CAD build for the part. Positions are in the model's coordinates, mm. Face numbers are marked on the shaded views. A direction names the side the tool comes from. Round coordinates to 2 decimals unless told otherwise and drop trailing zeros.
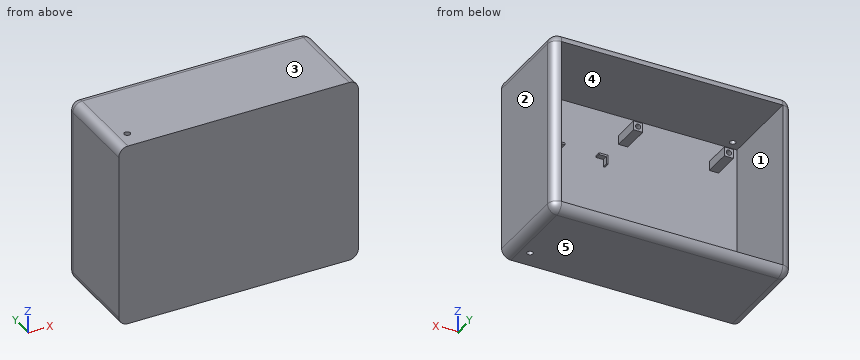
```python
from build123d import *

# Parameters (mm, degrees)
SKETCH1_W                                         = 130
SKETCH1_H                                         = 100
BOSS_EXTRUDE1_DEPTH                               = 51
SKETCH2_W                                         = 120
SKETCH2_H                                         = 90
CUT_EXTRUDE1_DEPTH                                = 46
FILLET2_R                                         = 5
FILLET4_R                                         = 5
SKETCH6_W                                         = 5
SKETCH6_H                                         = 5
BOSS_EXTRUDE2_DEPTH                               = 15
BOSS_EXTRUDE3_DEPTH                               = 3
F_4_CLEARANCE_HOLE2_D                             = 2.8448
F_4_CLEARANCE_HOLE2_DEPTH                         = 10
CSK_FOR_4_FLAT_HEAD_MACHINE_SCREW_100_D           = 3.2639
CSK_FOR_4_FLAT_HEAD_MACHINE_SCREW_100_DEPTH       = 10
CSK_FOR_4_FLAT_HEAD_MACHINE_SCREW_100_CSINK_D     = 5.715
CSK_FOR_4_FLAT_HEAD_MACHINE_SCREW_100_CSINK_ANGLE = 100
CSK_FOR_4_FLAT_HEAD_MACHINE_SCREW_100_TIP         = 0.980574487
CSK_FOR_4_FLAT_HEAD_MACHINE_SCREW_2_D             = 3.2639
CSK_FOR_4_FLAT_HEAD_MACHINE_SCREW_2_DEPTH         = 10
CSK_FOR_4_FLAT_HEAD_MACHINE_SCREW_2_CSINK_D       = 5.715
CSK_FOR_4_FLAT_HEAD_MACHINE_SCREW_2_CSINK_ANGLE   = 100
CSK_FOR_4_FLAT_HEAD_MACHINE_SCREW_2_TIP           = 0.980574487


# Some blends are built 0.0001 mm under size
with BuildPart() as part:
    # Sketch1 → Boss-Extrude1 (new body)
    with BuildSketch(Plane(origin=(0, 0, 0), x_dir=(1, 0, 0), z_dir=(0, 1, 0))):
        Rectangle(SKETCH1_W, SKETCH1_H)
    extrude(amount=BOSS_EXTRUDE1_DEPTH)

    # Sketch2 → Cut-Extrude1 (cut)
    with BuildSketch(Plane(origin=(0, 51, 0), x_dir=(1, 0, 0), z_dir=(0, 1, 0))):
        Rectangle(SKETCH2_W, SKETCH2_H)
    extrude(amount=-CUT_EXTRUDE1_DEPTH, mode=Mode.SUBTRACT)

    # Fillet2
    fillet2_edges = [part.edges().sort_by_distance(p)[0] for p in [
        (-65, 51, 0),
        (0, 51, 50),
        (65, 51, 0),
        (0, 51, -50),
    ]]
    fillet(fillet2_edges, radius=FILLET2_R - 0.0001)  # a hair under: the kernel refuses the full size

    # Fillet4
    # the kernel refuses this fillet: 5 mm, written as the material it takes off along each edge
    with BuildSketch(Plane(origin=(60, 51, 45), x_dir=(0, 0, 1), z_dir=(-1, 0, 0))) as fillet4_piece_1:
        with BuildLine():
            CenterArc((0.0001, -4.9999), 4.9999, 0, 90)
            Line((5, -4.9999), (5, 0))
            Line((5, 0), (0.0001, 0))
        make_face()
    revolve(axis=Axis((60, 51, 45), (0, 1, 0)), revolution_arc=90, mode=Mode.SUBTRACT)
    with BuildSketch(Plane(origin=(-60, 51, 45), x_dir=(-1, 0, 0), z_dir=(0, 0, -1))) as fillet4_piece_2:
        with BuildLine():
            CenterArc((0.0001, -4.9999), 4.9999, 0, 90)
            Line((5, -4.9999), (5, 0))
            Line((5, 0), (0.0001, 0))
        make_face()
    revolve(axis=Axis((-60, 51, 45), (0, 1, 0)), revolution_arc=90, mode=Mode.SUBTRACT)
    with BuildSketch(Plane(origin=(60, 51, -45), x_dir=(1, 0, 0), z_dir=(0, 0, 1))) as fillet4_piece_3:
        with BuildLine():
            CenterArc((0.0001, -4.9999), 4.9999, 0, 90)
            Line((5, -4.9999), (5, 0))
            Line((5, 0), (0.0001, 0))
        make_face()
    revolve(axis=Axis((60, 51, -45), (0, 1, 0)), revolution_arc=90, mode=Mode.SUBTRACT)
    with BuildSketch(Plane(origin=(-60, 51, -45), x_dir=(0, 0, -1), z_dir=(1, 0, 0))) as fillet4_piece_4:
        with BuildLine():
            CenterArc((0.0001, -4.9999), 4.9999, 0, 90)
            Line((5, -4.9999), (5, 0))
            Line((5, 0), (0.0001, 0))
        make_face()
    revolve(axis=Axis((-60, 51, -45), (0, 1, 0)), revolution_arc=90, mode=Mode.SUBTRACT)
    with BuildSketch(Plane(origin=(-65, -12.5, -50), x_dir=(1, 0, 0), z_dir=(0, 1, 0)), Plane(origin=(-65, -12.5, 50), x_dir=(0, 0, -1), z_dir=(0, 1, 0))) as fillet4_piece_5:
        with BuildLine():
            CenterArc((FILLET4_R, -FILLET4_R), FILLET4_R, 90, 90)
            Line((0, -FILLET4_R), (0, 0))
            Line((0, 0), (FILLET4_R, 0))
        make_face()
    extrude(amount=63.5, mode=Mode.SUBTRACT)
    with BuildSketch(Plane(origin=(65, -12.5, -50), x_dir=(-1, 0, 0), z_dir=(0, 1, 0)), Plane(origin=(65, -12.5, 50), x_dir=(0, 0, -1), z_dir=(0, 1, 0))) as fillet4_piece_6:
        with BuildLine():
            CenterArc((FILLET4_R, FILLET4_R), FILLET4_R, 180, 90)
            Line((0, FILLET4_R), (0, 0))
            Line((0, 0), (FILLET4_R, 0))
        make_face()
    extrude(amount=63.5, mode=Mode.SUBTRACT)

    # Sketch6 → Boss-Extrude2 (add)
    with BuildSketch(Plane(origin=(0, 5, 0), x_dir=(1, 0, 0), z_dir=(0, 1, 0))):
        with Locations((-47.5, 32.5)):
            Rectangle(SKETCH6_W, SKETCH6_H)
        with Locations((-47.5, -31.53)):
            Rectangle(SKETCH6_W, SKETCH6_H)
        with Locations((1.77, 32.5)):
            Rectangle(SKETCH6_W, SKETCH6_H)
        with Locations((1.77, -31.53)):
            Rectangle(SKETCH6_W, SKETCH6_H)
    extrude(amount=BOSS_EXTRUDE2_DEPTH)

    # Sketch9 → Boss-Extrude3 (add)
    with BuildSketch(Plane(origin=(0, 5, 0), x_dir=(1, 0, 0), z_dir=(0, 1, 0))):
        Polygon((11.5, -14.03), (11.5, -19.03), (16.5, -19.03), (16.5, -18.03), (12.5, -18.03), (12.5, -14.03), align=None)
        Polygon((11.5, 27.97), (16.5, 27.97), (16.5, 26.97), (12.5, 26.97), (12.5, 22.97), (11.5, 22.97), align=None)
        Polygon((40, 27.97), (40, 22.97), (39, 22.97), (39, 26.97), (35, 26.97), (35, 27.97), align=None)
        Polygon((40, -19.03), (35, -19.03), (35, -18.03), (39, -18.03), (39, -14.03), (40, -14.03), align=None)
    extrude(amount=BOSS_EXTRUDE3_DEPTH)

    # #4 Clearance Hole2
    with Locations(Plane(origin=(58.965440854, 20, -19.145321972), x_dir=(1, 0, 0), z_dir=(0, 1, 0))):
        with Locations((-106.465440854, -50.675321972), (-57.195440854, -50.675321972), (-57.195440854, 13.354678028), (-106.465440854, 13.354678028)):
            Hole(F_4_CLEARANCE_HOLE2_D / 2, depth=F_4_CLEARANCE_HOLE2_DEPTH)

    # CSK for _4 Flat Head Machine Screw _100
    with Locations(Plane(origin=(58.965440854, 7.381222334, 55), x_dir=(1, 0, 0), z_dir=(0, 0, 1))):
        with Locations((-113.965440854, 2.618777666)):
            CounterSinkHole(CSK_FOR_4_FLAT_HEAD_MACHINE_SCREW_100_D / 2, CSK_FOR_4_FLAT_HEAD_MACHINE_SCREW_100_CSINK_D / 2, depth=CSK_FOR_4_FLAT_HEAD_MACHINE_SCREW_100_DEPTH, counter_sink_angle=CSK_FOR_4_FLAT_HEAD_MACHINE_SCREW_100_CSINK_ANGLE)
            with Locations((0, 0, -(CSK_FOR_4_FLAT_HEAD_MACHINE_SCREW_100_DEPTH + CSK_FOR_4_FLAT_HEAD_MACHINE_SCREW_100_TIP / 2))):  # 118° drill point
                Cone(0, CSK_FOR_4_FLAT_HEAD_MACHINE_SCREW_100_D / 2, CSK_FOR_4_FLAT_HEAD_MACHINE_SCREW_100_TIP, mode=Mode.SUBTRACT)

    # CSK for _4 Flat Head Machine Screw _ 2
    with Locations(Plane(origin=(58.965440854, 7.381222334, -55), x_dir=(-1, 0, 0), z_dir=(0, 0, -1))):
        with Locations((3.965440854, 2.618777666)):
            CounterSinkHole(CSK_FOR_4_FLAT_HEAD_MACHINE_SCREW_2_D / 2, CSK_FOR_4_FLAT_HEAD_MACHINE_SCREW_2_CSINK_D / 2, depth=CSK_FOR_4_FLAT_HEAD_MACHINE_SCREW_2_DEPTH, counter_sink_angle=CSK_FOR_4_FLAT_HEAD_MACHINE_SCREW_2_CSINK_ANGLE)
            with Locations((0, 0, -(CSK_FOR_4_FLAT_HEAD_MACHINE_SCREW_2_DEPTH + CSK_FOR_4_FLAT_HEAD_MACHINE_SCREW_2_TIP / 2))):  # 118° drill point
                Cone(0, CSK_FOR_4_FLAT_HEAD_MACHINE_SCREW_2_D / 2, CSK_FOR_4_FLAT_HEAD_MACHINE_SCREW_2_TIP, mode=Mode.SUBTRACT)


solid = part.part
```
Item 1: 3-axis set-ups, long thin cutter, end or side, ignore diameter. For the marked faces 4 and 5: which of +Z, -Z, +X, -X, +Y, -Y reach the whole face in a straight line?
Answers follow:
face 4: +Y
face 5: -Z, +X, -X, +Y, -Y
Item 2: Flat gauge pins, fed straight in: P1, Ø4, axis at x = -47.5, z = 30.5, coming from the +Y side; P2, Ø1, axis at x = 26.5, z = -39, coming from the +Y side; P3, Ø2.5, axis at x = 1.77, z = -32.5, coming from the +Y side. Where does each tip first touch, or does it go through?
Answers follow:
P1: stops at y = 20
P2: stops at y = 5
P3: stops at y = 10
Item 3: Two-plate mould, pull along Z, no slides. Class the marked faces 1, 2 and 3: released by +Z, released by -Z, zero draft, split by the parting line, or undercut.
Answers follow:
face 1: undercut
face 2: zero draft
face 3: released by +Z
Item 4: Cut at A-A, the plane y = 14.5. State how many separate pieces and enclosed holes the cut face has, plus the area to 3 significant figures.
Answers follow:
separate pieces: 5
enclosed holes: 5
area: 2,250 mm2
Item 5: Probe line 1 (X direction, y = 13.5, z = -32.5); line 2 (Z direction, x = -47.5, y = 17.75); line 3 (Z direction, x = -51, y = 21). List the from-to ranges inside material, lowest first.
Answers follow:
line 1: x = -65 to -60, -50 to -48.92, -46.08 to -45, -0.73 to 0.35, 3.19 to 4.27, 60 to 65
line 2: z = -50 to -45, -35 to -33.92, -31.08 to -30, 29.03 to 30.11, 32.95 to 34.03, 45 to 50
line 3: z = -50 to -45, 45 to 50
